Model file for the job. Use its own axes, mm. Face numbers are marked on the shaded views. A direction names the side the tool comes from. Round coordinates to 2 decimals unless told otherwise and drop trailing zeros. Order: outer loops, then holes, each group sorted by start corner. A loop starts at its lowest first (then second) coordinate and runs counter-clockwise, first axis right, second up. Notation, with made-up numbers: (26.25, -38.5) -> (47.25, -38.5) arc R32 ccw to (47.25, -0.5) -> close; hole circle Ø3 at (13, -36). An arc over 180 degrees is marked (long way). Put each result on its own line as item: value. Start each with the question number.
Q1. Pull direction Y, two halves, no side cores. Call the marked faces 5, 6 and 7: released by +Y, released by -Y, zero draft, split by the parting line, or undercut.
Q2. 3-axis set-ups, long thin cutter, end or side, ignore diameter. For the marked faces 1, 2, 3 and 4: which of +Z, -Z, +X, -X, +Y, -Y reach the whole face in a straight line?
Q3. Cut at B-B, the plane x = 41. List the corners of the cut face in (y, z), and give its area (3 significant figures).
Q4. Cut at A-A, the plane x = 25. List the corners of the cut face in (y, z).
Q5. Cut at C-C, the plane y = 40.5. List the corners of the cut face in (x, z), and give its area (3 significant figures).
Q6. Flat gauge pins, fed straight in: P1, Ø5, axis at x = 25.5, z = 90, coming from the -Y side; P2, Ø14, axis at x = 28, z = 37.5, coming from the +Y side; P3, Ø8, axis at x = -14.5, z = 97.5, coming from the +Y side. Where does each tip first touch, or does it go through?
Q7. Probe L1, parallel to Y at x = 31.5, z = 26; L2, parallel to Y at x = -3.5, z = 62.5; L3, parallel to Y at x = -9, z = 113.5. List the from-to ranges inside material, lowest first.
from build123d import *

# Parameters (mm, degrees)
F1_DEPTH = 140


# Not quite as in the source:
# - ends of sketch curves that miss each other by under 0.0002 mm in the source are joined


with BuildPart() as f1:
    # F0 (on Top) → F1 (new body)
    with BuildSketch(Plane.XY):
        Polygon((9.8149545762, -17), (19.0525588833, -1), (37.5277626519, -1), (47.3427172281, 16), (38.1051129211, 32), (47.3427172281, 48), (37.5277626519, 65), (19.0525576719, 65), (9.8149545762, 81), (-9.8149545762, 81), (-19.0525576719, 65.0000020981), (-37.5277626519, 65), (-47.3427172281, 48), (-38.1051129211, 32), (-47.3427172281, 16), (-37.5277626519, -1), (-19.0525588833, -1), (-9.8149545762, -17), align=None)
        Polygon((-10.3923048454, 16), (-19.0525576719, 1.0000020981), (-36.3730621135, 1), (-45.0333161514, 16), (-36.3730621135, 31), (-19.0525540378, 31), align=None, mode=Mode.SUBTRACT)
        Polygon((-17.3205080757, 0), (-8.6602540378, 15), (8.6602540378, 15), (17.3205080757, 0), (8.6602540378, -15), (-8.6602540378, -15), align=None, mode=Mode.SUBTRACT)
        Polygon((8.6602540378, 17), (-8.6602540378, 17), (-17.3205080757, 32), (-8.9903810568, 46.4282032303), (-8.6602540378, 47), (8.6602540378, 47), (16.9903849907, 32.5717899559), (17.3205080757, 32), align=None, mode=Mode.SUBTRACT)
        Polygon((19.0525576719, 1.0000020981), (10.3923048454, 16), (14.7224318643, 23.5), (19.0525540378, 31), (36.3730621135, 31), (45.0333161514, 16), (36.3730621135, 1), align=None, mode=Mode.SUBTRACT)
        Polygon((-10.3923048454, 48), (-19.0525576719, 33.0000020981), (-36.3730621135, 33), (-45.0333161514, 48), (-36.3730621135, 63), (-19.0525540378, 63), align=None, mode=Mode.SUBTRACT)
        Polygon((19.0525576719, 33.0000020981), (10.3923048454, 48), (19.0525576719, 62.9999979019), (36.3730621135, 63), (45.0333161514, 48), (36.3730621135, 33), align=None, mode=Mode.SUBTRACT)
        Polygon((8.6602540378, 49), (-8.6602540378, 49), (-17.3205080757, 64), (-8.6602540378, 79), (8.6602540378, 79), (17.3205080757, 64), align=None, mode=Mode.SUBTRACT)
    extrude(amount=F1_DEPTH)


solid = f1.part
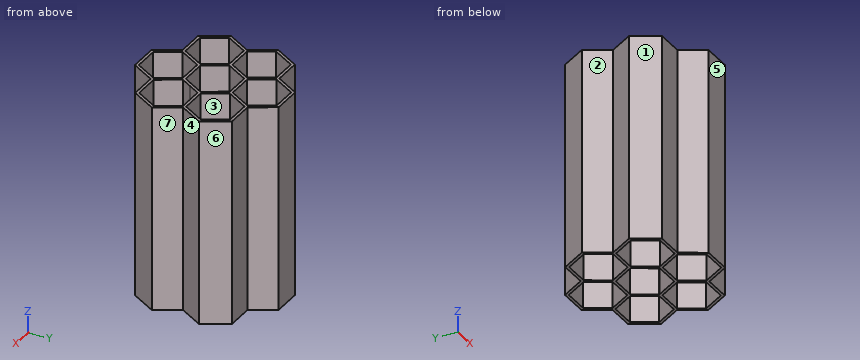
Ans:
1. face 5: released by -Y
1. face 6: released by +Y
1. face 7: undercut
2. face 1: +Z, -Z, -X, -Y
2. face 2: +Z, -Z, -X
2. face 3: +Z, -Z
2. face 4: +Z, -Z, +X
3. outline: (5.01, 0) -> (9.01, 0) -> (9.01, 140) -> (5.01, 140) -> close; (22.99, 0) -> (26.99, 0) -> (26.99, 140) -> (22.99, 140) -> close; (37.01, 0) -> (41.01, 0) -> (41.01, 140) -> (37.01, 140) -> close; (54.99, 0) -> (58.99, 0) -> (58.99, 140) -> (54.99, 140) -> close
3. area: 2,240 mm^2
4. outline: (-1, 0) -> (1, 0) -> (1, 140) -> (-1, 140) -> close; (31, 0) -> (33, 0) -> (33, 140) -> (31, 140) -> close; (63, 0) -> (65, 0) -> (65, 140) -> (63, 140) -> close
5. outline: (-43.01, 0) -> (-40.7, 0) -> (-40.7, 140) -> (-43.01, 140) -> close; (-14.72, 0) -> (-12.41, 0) -> (-12.41, 140) -> (-14.72, 140) -> close; (12.41, 0) -> (14.72, 0) -> (14.72, 140) -> (12.41, 140) -> close; (40.7, 0) -> (43.01, 0) -> (43.01, 140) -> (40.7, 140) -> close
5. area: 1,290 mm^2
6. P1: stops at y = -1
6. P2: stops at y = 65
6. P3: stops at y = 79.81
7. L1: y = -1 to 1, 31 to 33, 63 to 65
7. L2: y = -17 to -15, 15 to 17, 47 to 49, 79 to 81
7. L3: y = -17 to -14.41, 14.41 to 17.59, 46.41 to 49.59, 78.41 to 81
